CAD build for the part. Positions are in the model's coordinates, mm. A direction names the side the tool comes from. Give positions to 0.01 mm unless a question says otherwise; leave off trailing zeros. Loops run counter-clockwise (first coordinate to the right, second up) from the corner with the lowest first, then second, coordinate; pieces in that order, holes last. Notation, with made-up numbers: M -35.75,50.25 L -19.75,50.25 A35 ccw -19.75,83.25 Z; hole C 38,-29 d2. An arc over 180 degrees is marked long. Answer as CSV lines item,"result".
from build123d import *

# Parameters (mm, degrees)
SKETCH1_W                      = 20
SKETCH1_H                      = 41
BOSS_EXTRUDE1_DEPTH            = 10
BOSS_EXTRUDE1_2_DEPTH          = 10
SKETCH2_R                      = 1.5
CUT_EXTRUDE1_DEPTH             = 10
SKETCH3_R                      = 3
CUT_EXTRUDE2_DEPTH             = 3
SKETCH4_W                      = 8
SKETCH4_H                      = 41
BOSS_EXTRUDE2_DEPTH            = 35
SKETCH5_W                      = 62
SKETCH5_H                      = 41
BOSS_EXTRUDE3_DEPTH            = 15
CUT_EXTRUDE3_REACH             = 78.611
SKETCH6_R                      = 1.5
SKETCH7_R                      = 3
CUT_EXTRUDE4_DEPTH             = 3
SKETCH8_R                      = 12
CUT_EXTRUDE5_DEPTH             = 10
CUT_EXTRUDE6_REACH             = 78.611
SKETCH9_R                      = 6
CUT_EXTRUDE6_DIRECTION_2_DEPTH = 77.611030537
SKETCH10_R                     = 18.5
CUT_EXTRUDE7_DEPTH             = 8


with BuildPart() as part:
    # Sketch1 → Boss-Extrude1 (new body)
    with BuildSketch(Plane(origin=(0, 0, 0), x_dir=(1, 0, 0), z_dir=(0, 1, 0))):
        with Locations((33, 0)):
            Rectangle(SKETCH1_W, SKETCH1_H)
    extrude(amount=BOSS_EXTRUDE1_DEPTH)


with BuildPart() as body_2:
    # Sketch1 → Boss-Extrude1 2 (new body)
    with BuildSketch(Plane(origin=(0, 0, 0), x_dir=(1, 0, 0), z_dir=(0, 1, 0))):
        with Locations((-33, 0)):
            Rectangle(SKETCH1_W, SKETCH1_H)
    extrude(amount=BOSS_EXTRUDE1_2_DEPTH)


with BuildPart() as cut_extrude1_tool:
    # Sketch2 → Cut-Extrude1 (new body)
    with BuildSketch(Plane(origin=(0, 10, 0), x_dir=(1, 0, 0), z_dir=(0, 1, 0))):
        with Locations(Location((-38, 15.5, 0), (0, 0, 270))):
            Circle(SKETCH2_R)
        with Locations(Location((-38, -15.5, 0), (0, 0, 270))):
            Circle(SKETCH2_R)
        with Locations(Location((38, -15.5, 0), (0, 0, 270))):
            Circle(SKETCH2_R)
        with Locations(Location((38, 15.5, 0), (0, 0, 270))):
            Circle(SKETCH2_R)
    extrude(amount=-CUT_EXTRUDE1_DEPTH)


with BuildPart() as part_1:
    add(part.part)

    # Cut-Extrude1: cut by cut_extrude1_tool
    add(cut_extrude1_tool.part, mode=Mode.SUBTRACT)


with BuildPart() as body_2_1:
    add(body_2.part)

    # Cut-Extrude1: cut by cut_extrude1_tool
    add(cut_extrude1_tool.part, mode=Mode.SUBTRACT)


with BuildPart() as cut_extrude2_tool:
    # Sketch3 → Cut-Extrude2 (new body)
    with BuildSketch(Plane(origin=(0, 10, 0), x_dir=(1, 0, 0), z_dir=(0, 1, 0))):
        with Locations(Location((-38, 15.5, 0), (0, 0, 270))):
            Circle(SKETCH3_R)
        with Locations(Location((-38, -15.5, 0), (0, 0, 270))):
            Circle(SKETCH3_R)
        with Locations(Location((38, -15.5, 0), (0, 0, 270))):
            Circle(SKETCH3_R)
        with Locations(Location((38, 15.5, 0), (0, 0, 270))):
            Circle(SKETCH3_R)
    extrude(amount=-CUT_EXTRUDE2_DEPTH)


with BuildPart() as part_2:
    add(part_1.part)

    # Cut-Extrude2: cut by cut_extrude2_tool
    add(cut_extrude2_tool.part, mode=Mode.SUBTRACT)



with BuildPart() as body_2_2:
    add(body_2_1.part)

    # Cut-Extrude2: cut by cut_extrude2_tool
    add(cut_extrude2_tool.part, mode=Mode.SUBTRACT)


with BuildPart() as part_3:
    add(part_2.part)

    add(body_2_2.part)  # Boss-Extrude2 merges body 2
    # Sketch4 → Boss-Extrude2 (add)
    with BuildSketch(Plane(origin=(0, 10, 0), x_dir=(1, 0, 0), z_dir=(0, 1, 0))):
        with Locations((-27, 0)):
            Rectangle(SKETCH4_W, SKETCH4_H)
        with Locations((27, 0)):
            Rectangle(SKETCH4_W, SKETCH4_H)
    extrude(amount=BOSS_EXTRUDE2_DEPTH)

    # Sketch5 → Boss-Extrude3 (add)
    with BuildSketch(Plane(origin=(0, 45, 0), x_dir=(1, 0, 0), z_dir=(0, 1, 0))):
        Rectangle(SKETCH5_W, SKETCH5_H)
    extrude(amount=BOSS_EXTRUDE3_DEPTH)

    # Sketch6 → Cut-Extrude3 (cut, up to next)
    with BuildSketch(Plane(origin=(0, 60, 0), x_dir=(1, 0, 0), z_dir=(0, 1, 0)), mode=Mode.PRIVATE) as cut_extrude3_sk1:
        with Locations(Location((-14, 0, 0), (0, 0, 270))):
            Circle(SKETCH6_R)
    cut_extrude3_tool1 = extrude(cut_extrude3_sk1.sketch, amount=-CUT_EXTRUDE3_REACH, mode=Mode.PRIVATE) & part_3.part
    # Sketch6 → Cut-Extrude3 (cut, up to next)
    with BuildSketch(Plane(origin=(0, 60, 0), x_dir=(1, 0, 0), z_dir=(0, 1, 0)), mode=Mode.PRIVATE) as cut_extrude3_sk2:
        with Locations(Location((0, 14, 0), (0, 0, 270))):
            Circle(SKETCH6_R)
    cut_extrude3_tool2 = extrude(cut_extrude3_sk2.sketch, amount=-CUT_EXTRUDE3_REACH, mode=Mode.PRIVATE) & part_3.part
    # Sketch6 → Cut-Extrude3 (cut, up to next)
    with BuildSketch(Plane(origin=(0, 60, 0), x_dir=(1, 0, 0), z_dir=(0, 1, 0)), mode=Mode.PRIVATE) as cut_extrude3_sk3:
        with Locations(Location((14, 0, 0), (0, 0, 270))):
            Circle(SKETCH6_R)
    cut_extrude3_tool3 = extrude(cut_extrude3_sk3.sketch, amount=-CUT_EXTRUDE3_REACH, mode=Mode.PRIVATE) & part_3.part
    # Sketch6 → Cut-Extrude3 (cut, up to next)
    with BuildSketch(Plane(origin=(0, 60, 0), x_dir=(1, 0, 0), z_dir=(0, 1, 0)), mode=Mode.PRIVATE) as cut_extrude3_sk4:
        with Locations(Location((0, -14, 0), (0, 0, 270))):
            Circle(SKETCH6_R)
    cut_extrude3_tool4 = extrude(cut_extrude3_sk4.sketch, amount=-CUT_EXTRUDE3_REACH, mode=Mode.PRIVATE) & part_3.part
    add(cut_extrude3_tool1.solids().sort_by_distance((-14, 60, 0))[0], mode=Mode.SUBTRACT)
    add(cut_extrude3_tool2.solids().sort_by_distance((0, 60, -14))[0], mode=Mode.SUBTRACT)
    add(cut_extrude3_tool3.solids().sort_by_distance((14, 60, 0))[0], mode=Mode.SUBTRACT)
    add(cut_extrude3_tool4.solids().sort_by_distance((0, 60, 14))[0], mode=Mode.SUBTRACT)

    # Sketch7 → Cut-Extrude4 (cut)
    with BuildSketch(Plane.XZ.offset(-45)):
        with Locations(Location((0, 14, 0), (0, 0, 270))):
            Circle(SKETCH7_R)
        with Locations(Location((14, 0, 0), (0, 0, 270))):
            Circle(SKETCH7_R)
        with Locations(Location((0, -14, 0), (0, 0, 270))):
            Circle(SKETCH7_R)
        with Locations(Location((-14, 0, 0), (0, 0, 270))):
            Circle(SKETCH7_R)
    extrude(amount=-CUT_EXTRUDE4_DEPTH, mode=Mode.SUBTRACT)

    # Sketch8 → Cut-Extrude5 (cut)
    with BuildSketch(Plane(origin=(0, 60, 0), x_dir=(1, 0, 0), z_dir=(0, 1, 0))):
        with Locations(Location((0, 0, 0), (0, 0, 270))):
            Circle(SKETCH8_R)
    extrude(amount=-CUT_EXTRUDE5_DEPTH, mode=Mode.SUBTRACT)

    # Sketch9 → Cut-Extrude6 (cut, up to next)
    with BuildSketch(Plane(origin=(0, 60, 0), x_dir=(1, 0, 0), z_dir=(0, 1, 0)), mode=Mode.PRIVATE) as cut_extrude6_sk1:
        with Locations(Location((0, 0, 0), (0, 0, 270))):
            Circle(SKETCH9_R)
    cut_extrude6_tool1 = extrude(cut_extrude6_sk1.sketch, amount=-CUT_EXTRUDE6_REACH, mode=Mode.PRIVATE) & part_3.part
    add(cut_extrude6_tool1.solids().sort_by_distance((0, 60, 0))[0], mode=Mode.SUBTRACT)

    # Sketch9 → Cut-Extrude6 direction 2 (cut)
    with BuildSketch(Plane(origin=(0, 60, 0), x_dir=(1, 0, 0), z_dir=(0, 1, 0))):
        with Locations(Location((0, 0, 0), (0, 0, 270))):
            Circle(SKETCH9_R)
    extrude(amount=CUT_EXTRUDE6_DIRECTION_2_DEPTH, mode=Mode.SUBTRACT)

    # Sketch10 → Cut-Extrude7 (cut)
    with BuildSketch(Plane(origin=(0, 60, 0), x_dir=(1, 0, 0), z_dir=(0, 1, 0))):
        with Locations(Location((0, 0, 0), (0, 0, 270))):
            Circle(SKETCH10_R)
    extrude(amount=-CUT_EXTRUDE7_DEPTH, mode=Mode.SUBTRACT)


solid = part_3.part
1) Mould opens along X. For faces 1 (the face through (-1, 50, 20.5)), 2 (the face through (-31, 35, 0)), 3 (the face through (40.03, 8.52, 13.29)) say: +X half, -X half, draft (parallel to the pull), parting line (faces both ways), or undercut.
Answer below:
face 1,"draft"
face 2,"-X half"
face 3,"undercut"
2) Flat gauge pins, fed straight in: pin 1 (4 mm diameter, centred on x = -14, z = 0, fed in from -Y); pin 2 (3 mm diameter, centred on y = 48.5, z = 6.5, fed in from +X); pin 3 (5.5 mm diameter, centred on x = -38, z = 15.5, fed in from -Y); pin 4 (3.5 mm diameter, centred on x = 37.5, z = 8, fed in from +Y). Where does each tip first touch, or does it go through?
Answer below:
pin 1,"stops at y = 48"
pin 2,"stops at x = 31"
pin 3,"stops at y = 0"
pin 4,"stops at y = 10"
3) Which spindle directions (+Z, -Z, +X, -X, +Y, -Y) get a long thin tool onto all of the face, cutting with end or side? Do faces 4 (the face through (31, 35, 0)), 5 (the face through (37.1, 3.5, -16.7)), 6 (the face through (40.03, 8.52, -17.71)), 7 (the face through (23, 22, 0)), 8 (the face through (12.7, 48, -1.3)). Say none if no direction does.
Answer below:
face 4,"+Z, -Z, +X, +Y"
face 5,"+Y, -Y"
face 6,"+Y"
face 7,"+Z, -Z, -Y"
face 8,"-Y"
4) Band-saw the part on D-D on x = 0. Give the number of separate pieces and of enclosed holes in the cut face, and give its area (3 significant figures).
Answer below:
separate pieces,"4"
enclosed holes,"0"
area,"151 mm^2"
5) Band-saw the part on B-B on x = 38. Give the cut face in (y, z), and give its area (3 significant figures).
Answer below:
outline,"M 0,-20.5 L 10,-20.5 L 10,-18.5 L 7,-18.5 L 7,-17 L 0,-17 Z; M 0,-14 L 7,-14 L 7,-12.5 L 10,-12.5 L 10,12.5 L 7,12.5 L 7,14 L 0,14 Z; M 0,17 L 7,17 L 7,18.5 L 10,18.5 L 10,20.5 L 0,20.5 Z"
area,"332 mm^2"
6) Drill centre lines: line 1 (X direction, y = 41, z = -0.5); line 2 (X direction, y = 51, z = 0.5); line 3 (X direction, y = 56.5, z = 0). Where is each one in solid material? Low to high. Write a range as from..to.
Answer below:
line 1,"x = -31..-23, 23..31"
line 2,"x = -31..-15.41, -12.59..-11.99, 11.99..12.59, 15.41..31"
line 3,"x = -31..-18.5, 18.5..31"
7) Band-saw the part on A-A on y = 8.5. Give the cut face in (x, z), and give its area (3 significant figures).
Answer below:
outline,"M -43,-20.5 L -23,-20.5 L -23,20.5 L -43,20.5 Z; M 23,-20.5 L 43,-20.5 L 43,20.5 L 23,20.5 Z; hole C -38,-15.5 d6; hole C -38,15.5 d6; hole C 38,-15.5 d6; hole C 38,15.5 d6"
area,"1,530 mm^2"
8) Band-saw the part on C-C on y = 23.5. Give the cut face in (x, z).
Answer below:
outline,"M -31,-20.5 L -23,-20.5 L -23,20.5 L -31,20.5 Z; M 23,-20.5 L 31,-20.5 L 31,20.5 L 23,20.5 Z"
